Autodesk Inventor part; units mm, degrees
ref_plane "YZ Plane" through (0, 0, 0) normal (1, 0, 0) x (0, 1, 0)
ref_plane "XZ Plane" through (0, 0, 0) normal (0, 1, 0) x (-1, 0, 0)
ref_plane "XY Plane" through (0, 0, 0) normal (0, 0, 1) x (1, 0, 0)
sketch "スケッチ1" plane through (0, 0, 0) normal (0, 0, 1) x (1, 0, 0)
  circle A0 centre (0, 0) radius 50
  dimension "d0" = 100
extrude "押し出し1" add sketch "スケッチ1" along normal blind 2.5
sketch "スケッチ2" plane through (0, 0, 0) normal (0, 0, -1) x (-1, 0, 0)
  circle A0 centre (0, 0) radius 52
  dimension "d3" = 104
extrude "押し出し2" add sketch "スケッチ2" along normal blind 2.5
sketch "スケッチ3" plane through (0, 0, -2.5) normal (0, 0, -1) x (-1, 0, 0)
  point P0 (0, 0)
  point P1 (0, 0)
hole "穴1" at (0, 0, -2.5) direction (0, 0, 1) diameter 10 end through all
sketch "スケッチ4" plane through (0, 0, 2.5) normal (0, 0, 1) x (1, 0, 0)
  point P0 (0, 0)
  point P1 (0, 44)
  dimension "d13" = 44
hole "穴2" at (0, 44, 2.5) direction (0, 0, -1) diameter 10 end through all
pattern_circular "円形状パターン1" count 4 over 360 about axis through (0, 0, 144.6632) along (0, 0, -1) of "穴2"
sketch "スケッチ5" plane through (0, 0, -2.5) normal (0, 0, -1) x (-1, 0, 0)
  circle A0 centre (28.7245, 26.8039) radius 17.2489
  circle A1 centre (0, -44) radius 5
  circle A2 centre (0, 0) radius 44
  line L0 (31.1127, 31.1127) -> (0, 0)
  circle A3 centre (0, 44) radius 5
  line L1 (0, 0) -> (0, 44)
  dimension "d24" = 45
hole "穴3" at (-31.1127, 31.1127, -2.5) direction (0, 0, 1) diameter 4.2 end through all
pattern_circular "円形状パターン2" count 4 over 360 about axis through (0, 0, 0) along (0, 0, -1) of "穴3"
sketch "スケッチ6" plane through (0, 0, 2.5) normal (0, 0, 1) x (1, 0, 0)
  circle A0 centre (0, 0) radius 35
  circle A1 centre (0, 0) radius 15
  circle A2 centre (0, 25) radius 10
  circle A3 centre (-23.7764, 7.7254) radius 10
  circle A4 centre (-14.6946, -20.2254) radius 10
  circle A5 centre (14.6946, -20.2254) radius 10
  circle A6 centre (23.7764, 7.7254) radius 10
  dimension "d35" = 70
  dimension "d36" = 30
  dimension "d39" = 360
extrude "押し出し3" cut sketch "スケッチ6" against normal through all contours A6 | A5 | A2 | A4 | A3
properties part number "出力板" material "アルミニウム 6061"
Can you work these out from the model? Positions are in its coordinate system, mm. A direction names the side the tool comes from. Coordinates: 2 decimals unless noted, no trailing zeros. Order: outer loops, then holes, each group sorted by start corner. A loop starts at its lowest first (then second) coordinate and runs counter-clockwise, first axis right, second up. Notation, with made-up numbers: (-35.75, -25.75) -> (16.25, -25.75) arc R17 cw to (16.25, -6.75) -> close; hole circle Ø1 at (-13, 35). An arc over 180 degrees is marked (long way). Write each question's results on one line, items separated by ' | '.
Item 1: I want a section at C-C, the plane y = -22.5. Write out the boundary of the cut face in (x, z).
Results are:
outline: (-46.88, -2.5) -> (-24.43, -2.5) -> (-24.43, 2.5) -> (-44.65, 2.5) -> (-44.65, 0) -> (-46.88, 0) -> close; (-4.96, -2.5) -> (4.96, -2.5) -> (4.96, 2.5) -> (-4.96, 2.5) -> close; (24.43, -2.5) -> (46.88, -2.5) -> (46.88, 0) -> (44.65, 0) -> (44.65, 2.5) -> (24.43, 2.5) -> close
Item 2: I want a section at A-A, the plane x = -43.5. Write out the boundary of the cut face in (y, z), then the cut area to 3 significant figures.
Results are:
outline: (-28.49, -2.5) -> (-4.97, -2.5) -> (-4.97, 2.5) -> (-24.65, 2.5) -> (-24.65, 0) -> (-28.49, 0) -> close; (4.97, -2.5) -> (28.49, -2.5) -> (28.49, 0) -> (24.65, 0) -> (24.65, 2.5) -> (4.97, 2.5) -> close | area: 216 mm²
Item 3: I'm going to push flat-ended pins straight in: pin 1 Ø8 at (x, y) = (0, 44) entering from -Z; pin 2 Ø1.5 at (x, z) = (34, 2) entering from -Y; pin 3 Ø1 at (y, z) = (11.5, -1.5) entering from -X; pin 4 Ø3 at (x, z) = (1.5, 0.5) entering from +Y. Where does each tip first touch, or does it pass through?
Results are:
pin 1: through | pin 2: y = -37.34 | pin 3: x = -50.82 | pin 4: y = 52
Item 4: I want a section at B-B, the plane y = -44. Write out the boundary of the cut face in (x, z), then the cut area to 3 significant figures.
Results are:
outline: (-27.71, -2.5) -> (-5, -2.5) -> (-5, 2.5) -> (-23.75, 2.5) -> (-23.75, 0) -> (-27.71, 0) -> close; (5, -2.5) -> (27.71, -2.5) -> (27.71, 0) -> (23.75, 0) -> (23.75, 2.5) -> (5, 2.5) -> close | area: 207 mm²
Item 5: If I drill on line 1 along X through (y, z) = (-31, 2); line 2 along X through (y, z) = (-11.5, -0.7); line 3 along Y through (x, z) = (-2, -0.2), over which ranges is the centre line in solid material (lowest first)?
Results are:
line 1: -39.23 to -33.21, -29.02 to 29.02, 33.21 to 39.23 | line 2: -50.71 to -19.58, -9.81 to 9.81, 19.58 to 50.71 | line 3: -51.96 to -48.58, -39.42 to -4.58, 4.58 to 15.2, 34.8 to 39.42, 48.58 to 51.96
Item 6: Which directions (+Z, -Z, +X, -X, +Y, -Y) give clear straight access to the entire face, cutting with the end or side of a thin tool? Please do faces 5 (the face through (27, 43, 0)), 6 (the face through (0, 49, 0)).
Results are:
face 5: +Z | face 6: +Z, -Z
Item 7: I want a section at D-D, the plane z = 1. Count the separate pieces of the cut face and the enclosed holes in it, then the cut area to 3 significant figures.
Results are:
separate pieces: 1 | enclosed holes: 14 | area: 5,840 mm²
Item 8: If we mould it in two halves opening along Y, with no side actions, what happens to faces 1 (the face through (-1, -10, 2.5)), 2 (the face through (4.88, -1.08, 0.04)), 3 (the face through (30.839, 33.195, 0.035)), 4 (the face through (41.265, 31.641, -1.232))? For each: +Y half, -Y half, draft (parallel to the pull), parting line (faces both ways), or undercut.
Results are:
face 1: draft | face 2: undercut | face 3: undercut | face 4: parting line
